Can you work these out from the drawing? Everything is in mm from the part's minimum corner. Give positions to 0.01 mm unless a question says otherwise; leave off trailing zeros. Loops run counter-clockwise (first coordinate to the right, second up) from the corner with the lowest first, then second, coordinate; pieces in that order, holes last. Notation, with made-up numbers: M 26,10 L 47,10 A18 ccw 47,16 Z; hole C 68.5,-30 d1. An arc over 180 degrees is marked long. Use CSV: the item, a comma, the result in double quotes.
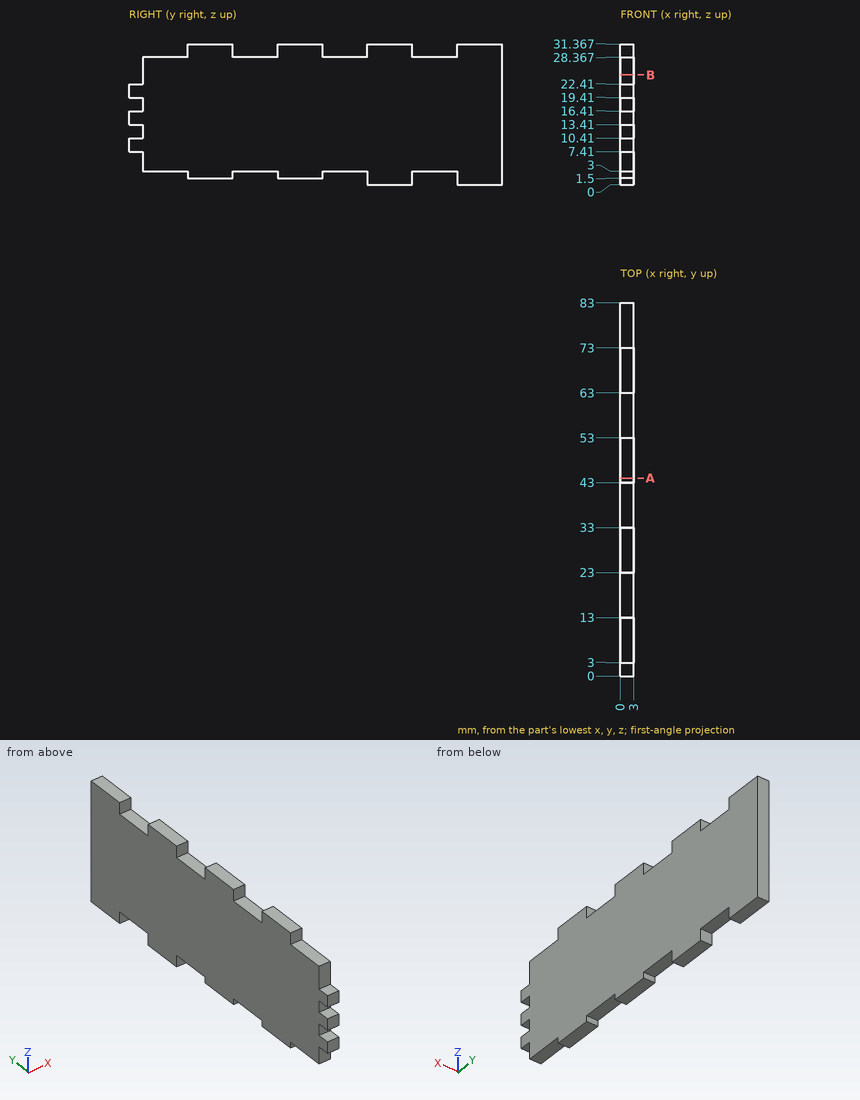
Q1. I want a section at A-A, the plane y = 44. Please give me the cut outline in (x, z).
Model answer:
outline,"M 0,3 L 3,3 L 3,28.37 L 0,28.37 Z"
Q2. I want a section at B-B, the plane z = 24.5. Please give me the cut outline in (x, y), then the cut area to 3 significant figures.
Model answer:
outline,"M 0,3 L 3,3 L 3,83 L 0,83 Z"
area,"240 mm2"
Q3. I'm going to push flat-ended pins straight in: P1, Ø3, axis at y = 22.5, z = 25, coming from the -X side; P2, Ø0.9, axis at x = 1, z = 29.5, coming from the -Y side; P3, Ø0.9, axis at x = 1.5, y = 26.5, coming from the -Z side; P4, Ø1, axis at x = 2.5, y = 15, coming from the -Z side. Where does each tip first touch, or does it pass through?
Model answer:
P1,"x = 0"
P2,"y = 13"
P3,"z = 3"
P4,"z = 1.5"
Q4. Please list where these lines run through material, in increasing order: L1, parallel to Y at x = 2.45, z = 17.5; L2, parallel to Z at x = 2.1, y = 64; L3, parallel to Z at x = 1.9, y = 16.5. Write a range as from..to.
Model answer:
L1,"3..83"
L2,"3..28.37"
L3,"1.5..31.37"
